Here's how the part is built. I have some questions about the finished solid (model axes, mm). Face numbers are marked on the shaded views. Coordinates: 2 decimals unless noted, no trailing zeros. Loops run counter-clockwise (first coordinate to the right, second up) from the corner with the lowest first, then second, coordinate; pieces in that order, holes last. Notation, with made-up numbers: (36, 48.5) - (71, 48.5) arc R5 ccw to (71, 56.5) - close; hole circle Ø6 at (50, 29). An arc over 180 degrees is marked (long way). Use a Markdown table: item, result.
Autodesk Inventor part; units mm, degrees
ref_plane "YZ Plane" through (0, 0, 0) normal (1, 0, 0) x (0, 1, 0)
ref_plane "XZ Plane" through (0, 0, 0) normal (0, 1, 0) x (-1, 0, 0)
ref_plane "XY Plane" through (0, 0, 0) normal (0, 0, 1) x (1, 0, 0)
sketch "Szkic1" plane through (0, 0, 0) normal (0, 0, 1) x (1, 0, 0)
  circle A0 centre (0, 0) radius 32.5
  circle A1 centre (0, 0) radius 32
  dimension "d0" = 65
  dimension "d1" = 64
extrude "Wyciągnięcie proste1" add sketch "Szkic1" along normal blind 72
sketch "Szkic2" plane through (0, 0, 72) normal (0, 0, 1) x (1, 0, 0)
  line L0 (0, 0) -> (-28, 0)
  line L1 (-28, 0) -> (-28, 15.4919)
  circle A0 centre (0, 0) radius 32
  line L2 (-28, 0) -> (-28, -16.5)
  circle A1 centre (0, 0) radius 32.5
  line L3 (-28, -16.5) -> (28, -16.5)
  line L4 (52.8927, -0.6882) -> (26.703, 44.9724)
  line L5 (26.703, 44.9724) -> (-31.7097, 42.3671)
  line L6 (-31.7097, 42.3671) -> (-48.5067, -13.9887)
  line L7 (-48.5067, -13.9887) -> (-28, -16.5)
  line L8 (28, -16.5) -> (52.8927, -0.6882)
  dimension "d4" = 28
extrude "Wyciągnięcie proste2" cut sketch "Szkic2" against normal blind 77 contours L2 A0 L1 | L1 A0 L3 L2 | A0 L2 A1 L3 | A0 L3 L2 | L7 L6 L5 L4 L8 A1
sketch "Szkic3" plane through (-27.4181, -16.5, 72) normal (0, 1, 0) x (1, 0, 0)
  line L0 (-0.5819, 0) -> (55.4181, 0)
  line L1 (-0.5819, 0) -> (-0.5819, 5)
  line L2 (-0.5819, 0) -> (-0.5819, 72)
  line L3 (-0.5819, 5) -> (0, 5)
  line L4 (0, 72) -> (0, 0)
  line L5 (0, 5) -> (0, 10)
  line L6 (0, 10) -> (-0.5819, 10)
  line L7 (-0.5819, 10) -> (-0.5819, 5)
  line L8 (-0.5819, 72) -> (55.4181, 72)
  line L9 (-0.5819, 72) -> (-0.5819, 67)
  line L10 (-0.5819, 67) -> (0, 67)
  line L11 (0, 67) -> (0, 62)
  line L12 (0, 62) -> (-0.5819, 62)
  line L13 (-0.5819, 62) -> (-0.5819, 67)
  line L14 (55.4181, 72) -> (55.4181, 67)
  line L15 (55.4181, 72) -> (55.4181, 0)
  line L16 (55.4181, 67) -> (54.8361, 67)
  line L17 (54.8361, 0) -> (54.8361, 72)
  line L18 (54.8361, 67) -> (54.8361, 62)
  line L19 (54.8361, 62) -> (55.4181, 62)
  line L20 (55.4181, 62) -> (55.4181, 67)
  line L21 (55.4181, 0) -> (55.4181, 5)
  line L22 (55.4181, 5) -> (54.8361, 5)
  line L23 (54.8361, 5) -> (54.8361, 10)
  line L24 (54.8361, 10) -> (55.4181, 10)
  line L25 (55.4181, 10) -> (55.4181, 5)
  point P0 (27.4181, 72)
  point P1 (-0.5819, 62)
  point P2 (0, 62)
  point P3 (0, 67)
  point P4 (-0.5819, 67)
  dimension "d7" = 5
  dimension "d8" = 5
  dimension "d9" = 5
  dimension "d10" = 5
  dimension "d11" = 5
  dimension "d12" = 5
  dimension "d13" = 5
  dimension "d14" = 5
extrude "Wyciągnięcie proste3" add sketch "Szkic3" along normal blind 5 contours L2 L6 L4 L3 | L17 L24 L15 L22 | L2 L10 L4 L12 | L17 L16 L15 L19
sketch "Szkic4" plane through (28, -16.5, 62) normal (1, 0, 0) x (0, 0, -1)
  line L0 (52, 0) -> (52, 5)
  line L1 (57, 0) -> (57, 5)
  line L2 (52, 0) -> (57, 5)
  line L3 (57, 5) -> (52, 5)
  line L4 (57, 5) -> (52, 5)
  line L5 (52, 5) -> (57, 0)
  line L6 (0, 0) -> (-5, 0)
  line L7 (-5, 5) -> (0, 5)
  line L8 (-5, 0) -> (0, 5)
  line L9 (0, 5) -> (-5, 5)
  line L10 (-5, 5) -> (0, 0)
  circle A0 centre (-2.5, 2.5) radius 1.5
  circle A1 centre (54.5, 2.5) radius 1.5
  point P0 (62, 16.5)
  dimension "d17" = 3
  dimension "d18" = 3
extrude "Wyciągnięcie proste4" cut sketch "Szkic4" against normal up to surface (56 mm away) contours A1 L5 L2 | L2 L5 A1 | A1 L2 L5 | L2 A1 L5 | A0 L8 L10 | L10 L8 A0 | A0 L10 L8 | L10 A0 L8
properties part number "Obudowa, mniejsza"
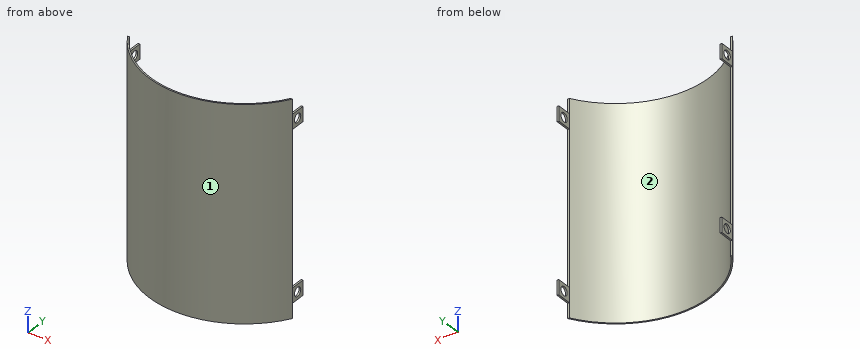
Q1. I want a section at D-D, the plane z = 56.5. Write out the boundary of the cut face in (x, y), then the cut area to 3 significant figures.
Check values:
| item | result |
|---|---|
| outline | (-28, -16.5) arc R32.5 ccw to (28, -16.5) - (27.42, -16.5) arc R32 cw to (-27.42, -16.5) - close |
| area | 33.3 mm^2 |
Q2. Will these pins go through, and if not, where does the flat tip stop? P1, Ø2, axis at x = -5, z = 12, coming from the +Y side; P2, Ø12, axis at y = -25, z = 59.5, coming from the +X side; P3, Ø10, axis at x = 10.5, z = 51, coming from the -Y side.
Check values:
| item | result |
|---|---|
| P1 | y = -31.43 |
| P2 | x = 26.37 |
| P3 | y = -32.03 |
Q3. If we mould it in two halves opening along X, with no side actions, what happens to the marked faces 1 and 2? For each: pulls with the +X half, pulls with the -X half, needs draft (parallel to the pull), parting line crosses it, or undercut.
Check values:
| item | result |
|---|---|
| face 1 | parting line crosses it |
| face 2 | undercut |
Q4. I want a section at A-A, the plane y = -14. Give the number of separate pieces and of enclosed holes in the cut face, then the cut area to 3 significant figures.
Check values:
| item | result |
|---|---|
| separate pieces | 8 |
| enclosed holes | 0 |
| area | 4.66 mm^2 |
Q5. I want a section at C-C, the plane y = -29.25. Write out the boundary of the cut face in (x, z).
Check values:
| item | result |
|---|---|
| outline | (-14.17, 0) - (-12.98, 0) - (-12.98, 72) - (-14.17, 72) - close; (12.98, 0) - (14.17, 0) - (14.17, 72) - (12.98, 72) - close |
Q6. Please list where these lines run through material, in increasing order: L1, parallel to Z at x = 27.75, y = -14; L2, parallel to X at y = -14.25, z = 5.5; L3, parallel to X at y = -25.75, z = 12.5. Write a range as from..to.
Check values:
| item | result |
|---|---|
| L1 | 5..6, 9..10, 62..63, 66..67 |
| L2 | -28..-27.42, 27.42..28 |
| L3 | -19.83..-19, 19..19.83 |
